Design review of the part built by this model. Coordinates are the model's own, in mm. A direction names the side the tool comes from. Give positions to 0.01 mm unless a question says otherwise; leave off trailing zeros. Loops run counter-clockwise (first coordinate to the right, second up) from the corner with the lowest first, then second, coordinate; pieces in that order, holes last. Notation, with made-up numbers: M 87,-15 L 114,-15 A20 ccw 114,22 Z; hole C 29,12 d3. An arc over 180 degrees is marked long. Use a Markdown table: item, result. Add a question column.
(1) Draft analysis for pull direction X (two halves, no side actions). For faces 1 (the face through (-39, 3, -30.48)), 2 (the face through (-0.905, 8.57, -15.071)), 3 (the face through (-38, 1, -29.21)), state which applies: pulls with the +X half, pulls with the -X half, needs draft (parallel to the pull), parting line crosses it, or undercut.
(2) For probe 1 along Z at (x, y) = (-51.5, 4); probe 2 along X at (y, z) = (5.75, -12); probe 3 along Z at (x, y) = (-10.5, 1), list the stretches that pass through material, from the lowest coordinate up.
(3) Add section C-C, the plane z = -13.5. Give the boundary of the cut face in (x, y) (3 decimals), then the cut area to 3 significant figures.
(4) For faces 4 (the face through (-75.29, 3.22, -0.95)), 5 (the face through (-74.387, 0.626, -28.637)), list the 3-axis set-ups (+Z, -Z, +X, -X, +Y, -Y) from which the entire face can be reached by the end or side of a thin tool; tool diameter is ignored.
(5) Add section A-A, the plane y = 3.75. Give the boundary of the cut face in (x, z) (3 decimals).
(6) Add section B-B, the plane x = -61.5. Give the boundary of the cut face in (y, z) (3 decimals).
(7) Add section D-D, the plane y = 8.75. Give the boundary of the cut face in (x, z) (3 decimals).
(8) Insertion check: pin 1 Ø2 at (x, z) = (-8, -26) entering from -Y (3 decimals); pin 2 Ø1.4 at (x, y) = (-34.5, 0.5) entering from +Z. Each pin has a flat end and moves straight along its axis. Give the tip position at first contact, or say it passes through.
Autodesk Inventor part; units mm, degrees
ref_plane "YZ Plane" through (0, 0, 0) normal (1, 0, 0) x (0, 1, 0)
ref_plane "XZ Plane" through (0, 0, 0) normal (0, 1, 0) x (-1, 0, 0)
ref_plane "XY Plane" through (0, 0, 0) normal (0, 0, 1) x (1, 0, 0)
sketch "Sketch1" plane through (0, 0, 0) normal (0, 1, 0) x (-1, 0, 0)
  line L0 (0, 0) -> (76.2, 0)
  line L1 (76.2, 0) -> (76.2, -30.48)
  line L2 (76.2, -30.48) -> (0, -30.48)
  line L3 (0, -30.48) -> (0, 0)
  dimension "d0" = 76.2
  dimension "d1" = 30.48
extrude "Extrusion1" add sketch "Sketch1" along normal blind 9.525
fillet "Fillet1" radius 3.175 8 edges at (0, 4.7625, 0) (0, 9.525, -15.24) (-38.1, 9.525, 0) (-38.1, 9.525, -30.48) (0, 4.7625, -30.48) (-76.2, 4.7625, 0) (-76.2, 9.525, -15.24) (-76.2, 4.7625, -30.48)
shell "Shell1" thickness 2.54 removed faces 1 at (-26.4583, 0, -20.32)
sketch "Sketch2" plane through (0, 0, 0) normal (0, -1, 0) x (1, 0, 0)
  line L0 (0, -27.305) -> (0, -3.175)
  arc A0 (-3.175, -30.48) -> (0, -27.305) centre (-3.175, -27.305) ccw
  line L1 (-73.025, -30.48) -> (-3.175, -30.48)
  arc A1 (0, -3.175) -> (-3.175, 0) centre (-3.175, -3.175) ccw
  line L2 (-3.175, 0) -> (-73.025, 0)
  arc A2 (-73.025, 0) -> (-76.2, -3.175) centre (-73.025, -3.175) ccw
  line L3 (-76.2, -3.175) -> (-76.2, -27.305)
  arc A3 (-76.2, -27.305) -> (-73.025, -30.48) centre (-73.025, -27.305) ccw
  arc A4 (-73.025, -1.27) -> (-74.93, -3.175) centre (-73.025, -3.175) ccw
  line L4 (-73.025, -1.27) -> (-3.175, -1.27)
  arc A5 (-1.27, -3.175) -> (-3.175, -1.27) centre (-3.175, -3.175) ccw
  line L5 (-1.27, -3.175) -> (-1.27, -27.305)
  arc A6 (-3.175, -29.21) -> (-1.27, -27.305) centre (-3.175, -27.305) ccw
  line L6 (-3.175, -29.21) -> (-73.025, -29.21)
  arc A7 (-74.93, -27.305) -> (-73.025, -29.21) centre (-73.025, -27.305) ccw
  line L7 (-74.93, -27.305) -> (-74.93, -3.175)
  point P0 (0, 0)
  dimension "d6" = 1.27
extrude "Extrusion2" cut sketch "Sketch2" against normal blind 1.27 contours L4 A5 L5 A6 L6 A7 L7 A4
properties part number "box_top"
Established:
| question | item | result |
|---|---|---|
| 1 | face 1 | needs draft |
| 1 | face 2 | pulls with the +X half |
| 1 | face 3 | undercut |
| 2 | probe 1 | -30.48 to -27.94, -2.54 to 0 |
| 2 | probe 2 | -76.2 to -73.66, -2.54 to 0 |
| 2 | probe 3 | -30.48 to -29.21, -1.27 to 0 |
| 3 | outline | M -76.2,0 L -74.93,0 L -74.93,1.27 L -73.66,1.27 L -73.66,6.35 A0.635 cw -73.025,6.985 L -3.175,6.985 A0.635 cw -2.54,6.35 L -2.54,1.27 L -1.27,1.27 L -1.27,0 L 0,0 L 0,6.35 A3.175 ccw -3.175,9.525 L -73.025,9.525 A3.175 ccw -76.2,6.35 Z |
| 3 | area | 222 mm^2 |
| 4 | face 4 | +Z, -X, +Y, -Y |
| 4 | face 5 | -Y |
| 5 | outline | M -76.2,-27.305 A3.175 ccw -73.025,-30.48 L -3.175,-30.48 A3.175 ccw 0,-27.305 L 0,-3.175 A3.175 ccw -3.175,0 L -73.025,0 A3.175 ccw -76.2,-3.175 Z; hole M -73.66,-27.305 A0.635 ccw -73.025,-27.94 L -3.175,-27.94 A0.635 ccw -2.54,-27.305 L -2.54,-3.175 A0.635 ccw -3.175,-2.54 L -73.025,-2.54 A0.635 ccw -73.66,-3.175 Z |
| 6 | outline | M 0,-30.48 L 6.35,-30.48 A3.175 ccw 9.525,-27.305 L 9.525,-3.175 A3.175 ccw 6.35,0 L 0,0 L 0,-1.27 L 1.27,-1.27 L 1.27,-2.54 L 6.35,-2.54 A0.635 cw 6.985,-3.175 L 6.985,-27.305 A0.635 cw 6.35,-27.94 L 1.27,-27.94 L 1.27,-29.21 L 0,-29.21 Z |
| 7 | outline | M -75.104,-27.305 A2.079 ccw -73.025,-29.384 L -3.175,-29.384 A2.079 ccw -1.096,-27.305 L -1.096,-3.175 A2.079 ccw -3.175,-1.096 L -73.025,-1.096 A2.079 ccw -75.104,-3.175 Z |
| 8 | pin 1 | y = 6.985 |
| 8 | pin 2 | z = 0 |
